```python
from build123d import *

# Parameters (mm, degrees)
SKETCH1_R           = 2.449
BOSS_EXTRUDE1_DEPTH = 2
BOSS_EXTRUDE2_START = 61.5600102
BOSS_EXTRUDE2_DEPTH = 61.5600102


with BuildPart() as part:
    # Sketch1 → Boss-Extrude1 (new body)
    with BuildSketch(Plane(origin=(0, 7e-09, 33.21323041), x_dir=(-1, 0, 0), z_dir=(0, -2.14626958308228e-10, -1.0))):
        with BuildLine():
            Line((-81.739723186, 76.765508674), (-70.033136805, 76.765508674))
            Line((-70.033136805, 76.765508674), (-9.168561928, 76.76533218))
            Line((-9.168561928, 76.76533218), (2.715276814, 76.76533218))
            ThreePointArc((2.715276814, 76.76533218), (5.543703939, 75.593759305), (6.715276814, 72.76533218))
            Line((6.715276814, 72.76533218), (6.715276814, 40.456513609))
            Line((6.715276814, 40.456513609), (6.715276814, 38.856513609))
            Line((6.715276814, 38.856513609), (6.715276814, 32.856513609))
            ThreePointArc((6.715276814, 32.856513609), (5.543703939, 30.028086484), (2.715276814, 28.856513609))
            Line((2.715276814, 28.856513609), (-81.739723186, 28.856513609))
            ThreePointArc((-81.739723186, 28.856513609), (-84.56815031, 30.028086484), (-85.739723186, 32.856513609))
            Line((-85.739723186, 32.856513609), (-85.739723186, 38.856513609))
            Line((-85.739723186, 38.856513609), (-85.739723186, 40.456513609))
            Line((-85.739723186, 40.456513609), (-85.739723186, 72.765508674))
            ThreePointArc((-85.739723186, 72.765508674), (-84.56815031, 75.593935798), (-81.739723186, 76.765508674))
        make_face()
        with Locations(Location((-2.764563873, 57.52531361, 0), (0, 0, 90))):
            Circle(SKETCH1_R, mode=Mode.SUBTRACT)
        with Locations(Location((-76.437246444, 57.525527244, 0), (0, 0, 90))):
            Circle(SKETCH1_R, mode=Mode.SUBTRACT)
        with BuildLine():
            Line((-63.603943309, 45.46049003), (-60.552841344, 45.460481183))
            Line((-60.552841344, 45.460481183), (-18.649041914, 45.460359671))
            Line((-18.649041914, 45.460359671), (-15.597940144, 45.460350824))
            ThreePointArc((-15.597940144, 45.460350824), (-12.365044057, 46.799449246), (-11.025926886, 50.032337566))
            Line((-11.025926886, 50.032337566), (-11.02588343, 65.018337566))
            ThreePointArc((-11.02588343, 65.018337566), (-12.364981852, 68.251233653), (-15.597870172, 69.590350824))
            Line((-15.597870172, 69.590350824), (-18.648972138, 69.59035918))
            Line((-18.648972138, 69.59035918), (-37.600871755, 69.590414358))
            Line((-37.600871755, 69.590414358), (-37.600871755, 70.340426004))
            Line((-37.600871755, 70.340426004), (-41.600871755, 70.340426004))
            Line((-41.600871755, 70.340426004), (-41.600871755, 69.590426004))
            Line((-41.600871755, 69.590426004), (-60.552771373, 69.590481183))
            Line((-60.552771373, 69.590481183), (-63.603873338, 69.59049003))
            ThreePointArc((-63.603873338, 69.59049003), (-66.836769424, 68.251391608), (-68.175886596, 65.018503288))
            Line((-68.175886596, 65.018503288), (-68.175930051, 50.032503288))
            ThreePointArc((-68.175930051, 50.032503288), (-66.83683163, 46.799607201), (-63.603943309, 45.46049003))
        make_face(mode=Mode.SUBTRACT)
    extrude(amount=BOSS_EXTRUDE1_DEPTH)

    # Sketch2 → Boss-Extrude2 (add)
    with BuildSketch(Plane.XY.offset(33.21323041).offset(BOSS_EXTRUDE2_START)):
        with BuildLine():
            Line((81.739723186, 28.856513609), (-2.715276814, 28.856513609))
            ThreePointArc((-2.715276814, 28.856513609), (-5.543703939, 30.028086484), (-6.715276814, 32.856513609))
            Line((-6.715276814, 32.856513609), (-6.715276814, 72.76533218))
            ThreePointArc((-6.715276814, 72.76533218), (-5.543703939, 75.593759305), (-2.715276814, 76.76533218))
            Line((-2.715276814, 76.76533218), (9.168561928, 76.76533218))
            Line((9.168561928, 76.76533218), (70.033136805, 76.765508674))
            Line((70.033136805, 76.765508674), (81.739723186, 76.765508674))
            ThreePointArc((81.739723186, 76.765508674), (84.56815031, 75.593935798), (85.739723186, 72.765508674))
            Line((85.739723186, 72.765508674), (85.739723186, 32.856513609))
            ThreePointArc((85.739723186, 32.856513609), (84.56815031, 30.028086484), (81.739723186, 28.856513609))
        make_face()
        with BuildLine():
            Line((9.168568018, 74.66533218), (70.033142895, 74.665508674))
            Line((70.033142895, 74.665508674), (81.739723186, 74.665508674))
            ThreePointArc((81.739723186, 74.665508674), (83.08322607, 74.109011558), (83.639723186, 72.765508674))
            Line((83.639723186, 72.765508674), (83.639723186, 32.856513609))
            ThreePointArc((83.639723186, 32.856513609), (83.08322607, 31.513010725), (81.739723186, 30.956513609))
            Line((81.739723186, 30.956513609), (-2.715276814, 30.956513609))
            ThreePointArc((-2.715276814, 30.956513609), (-4.058779699, 31.513010725), (-4.615276814, 32.856513609))
            Line((-4.615276814, 32.856513609), (-4.615276814, 72.76533218))
            ThreePointArc((-4.615276814, 72.76533218), (-4.058779699, 74.108835065), (-2.715276814, 74.66533218))
            Line((-2.715276814, 74.66533218), (9.168568018, 74.66533218))
        make_face(mode=Mode.SUBTRACT)
    extrude(amount=-BOSS_EXTRUDE2_DEPTH)


solid = part.part
```
Verification items for the finished model (mm, model axes). A direction names the side the tool comes from. Give positions to 0.01 mm unless a question says otherwise; leave off trailing zeros. Order: outer loops, then holes, each group sorted by start corner. A loop starts at its lowest first (then second) coordinate and runs counter-clockwise, first axis right, second up. Notation, with made-up numbers: (80.5, 44) - (136.5, 44) arc R19 ccw to (136.5, 63) - close; hole circle Ø5 at (57.25, -21). An arc over 180 degrees is marked (long way). Answer as CSV lines item,"result". Start each with the question number.
Item 1: Mould release check, pull along X, two halves, no side actions. Record for faces 4 (the face through (83.07, 74.12, 64.42)), 5 (the face through (74.046, 56.995, 32.227)), 6 (the face through (40, 30, 94.773)), 7 (the face through (85.74, 53, 63)): released by +X, released by -X, zero draft, split by the parting line, or undercut.
Item 2: Access from +Z, -Z, +X, -X, +Y, -Y to the whole of each face (thin tool, end or side, straight path). Record for faces 1 (the face through (39, 42, 31.213)), 2 (the face through (40, 30.957, 64)), 3 (the face through (66.8, 68.29, 32.23)).
Item 3: Section check D-D, the plane y = 42. Record the boundary of the cut face in (x, z), plus the area to 3 significant figures.
Item 4: Section check C-C, the plane x = 30.5. Record the boundary of the cut face in (y, z).
Item 5: Section check B-B, the plane z = 82. Record the boundary of the cut face in (x, y), plus the area to 3 significant figures.
Item 6: Section check A-A, the plane y = 54. Record the boundary of the cut face in (x, z), plus the area to 3 significant figures.
Item 7: Material ranges on L1, parallel to X at y = 64, z = 76.5; L2, parallel to Y at x = 80.5, z = 35; L3, parallel to Z at x = 46.5, y = 40, recorded low to high.
Filled in:
1,face 4,"undercut"
1,face 5,"undercut"
1,face 6,"zero draft"
1,face 7,"released by +X"
2,face 1,"-Z, +X, -X, +Y, -Y"
2,face 2,"+Z"
2,face 3,"+Z, -Z"
3,outline,"(-6.72, 31.21) - (85.74, 31.21) - (85.74, 94.77) - (83.64, 94.77) - (83.64, 33.21) - (-4.62, 33.21) - (-4.62, 94.77) - (-6.72, 94.77) - close"
3,area,"443 mm^2"
4,outline,"(28.86, 31.21) - (45.46, 31.21) - (45.46, 33.21) - (30.96, 33.21) - (30.96, 94.77) - (28.86, 94.77) - close; (69.59, 31.21) - (76.77, 31.21) - (76.77, 94.77) - (74.67, 94.77) - (74.67, 33.21) - (69.59, 33.21) - close"
5,outline,"(-6.72, 32.86) arc R4 ccw to (-2.72, 28.86) - (81.74, 28.86) arc R4 ccw to (85.74, 32.86) - (85.74, 72.77) arc R4 ccw to (81.74, 76.77) - (70.03, 76.77) - (9.17, 76.77) - (-2.72, 76.77) arc R4 ccw to (-6.72, 72.77) - close; hole (-4.62, 32.86) arc R1.9 ccw to (-2.72, 30.96) - (81.74, 30.96) arc R1.9 ccw to (83.64, 32.86) - (83.64, 72.77) arc R1.9 ccw to (81.74, 74.67) - (70.03, 74.67) - (9.17, 74.67) - (-2.72, 74.67) arc R1.9 ccw to (-4.62, 72.77) - close"
5,area,"561 mm^2"
6,outline,"(-6.72, 31.21) - (11.03, 31.21) - (11.03, 33.21) - (-4.62, 33.21) - (-4.62, 94.77) - (-6.72, 94.77) - close; (68.18, 31.21) - (85.74, 31.21) - (85.74, 94.77) - (83.64, 94.77) - (83.64, 33.21) - (68.18, 33.21) - close"
6,area,"329 mm^2"
7,L1,"-6.72 to -4.62, 83.64 to 85.74"
7,L2,"28.86 to 30.96, 74.67 to 76.77"
7,L3,"31.21 to 33.21"
